```python
from build123d import *

# Parameters (mm, degrees)
BOSS_EXTRUDE1_DEPTH = 6.35
CUT_EXTRUDE1_DEPTH  = 135.362158735
SKETCH3_R           = 1.4732
CUT_EXTRUDE2_DEPTH  = 135.362158735


with BuildPart() as part:
    # Sketch1 → Boss-Extrude1 (new body)
    with BuildSketch(Plane(origin=(0, 0, 0), x_dir=(1, 0, 0), z_dir=(0, 1, 0))):
        with BuildLine():
            Line((0, 0), (114.3, 0))
            ThreePointArc((114.3, 0), (116.096051224, -0.743948776), (116.84, -2.54))
            Line((116.84, -2.54), (116.84, -66.04))
            Line((116.84, -66.04), (97.79, -66.04))
            Line((97.79, -66.04), (97.79, -19.05))
            Line((97.79, -19.05), (0, -19.05))
            Line((0, -19.05), (0, 0))
        make_face()
    extrude(amount=BOSS_EXTRUDE1_DEPTH)

    # Sketch2 → Cut-Extrude1 (cut, through all)
    with BuildSketch(Plane(origin=(0, 6.35, 0), x_dir=(1, 0, 0), z_dir=(0, 1, 0))):
        Polygon((14.533087105, -12.7), (16.366174209, -9.525), (14.533087105, -6.35), (10.866912895, -6.35), (9.033825791, -9.525), (10.866912895, -12.7), align=None)
    extrude(amount=-CUT_EXTRUDE1_DEPTH, mode=Mode.SUBTRACT)

    # Sketch3 → Cut-Extrude2 (cut, through all)
    with BuildSketch(Plane.XZ):
        with Locations(Location((110.49, 38.1, 0), (0, 0, 270))):
            Circle(SKETCH3_R)
        with Locations(Location((110.49, 12.7, 0), (0, 0, 270))):
            Circle(SKETCH3_R)
    extrude(amount=-CUT_EXTRUDE2_DEPTH, mode=Mode.SUBTRACT)


solid = part.part
```
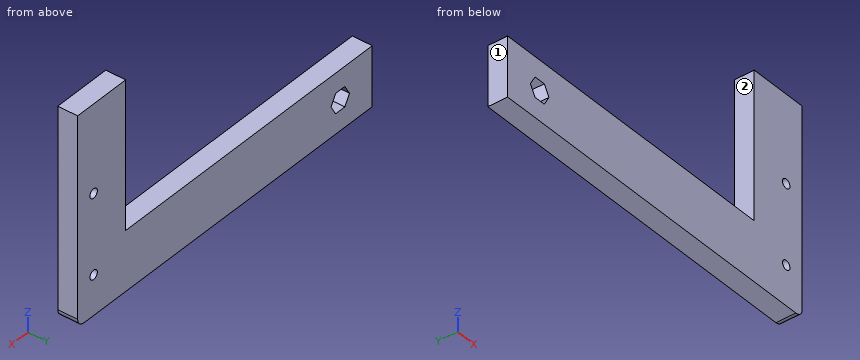
Source: CAD feature listing. Evaluate the final solid. Frame: model axes, mm. Face numbers are marked on the shaded views. A direction names the side the tool comes from. Give positions to 0.01 mm unless a question says otherwise; leave off trailing zeros. Order: outer loops, then holes, each group sorted by start corner. A loop starts at its lowest first (then second) coordinate and runs counter-clockwise, first axis right, second up. Notation, with made-up numbers: (4.5, 8.25) -> (60.5, 8.25) arc R10 ccw to (60.5, 18.25) -> close; hole circle Ø11 at (-5.5, 81). An arc over 180 degrees is marked (long way). Use a Markdown table: item, result.
Q1. First-contact query: P1, Ø3, axis at x = 30.5, y = 3.5, coming from the +Z side. Flat tip, straight axial feed; report the tip coordinate or a pass-through.
A:
| item | result |
|---|---|
| P1 | z = 19.05 |
Q2. Material intervals for line 1 (Z direction, x = 110.49, y = 2.25); line 2 (X direction, y = 5, z = 38.1); line 3 (Z direction, x = 18.5, y = 3), sorted ascending. Write a range as [from, to].
A:
| item | result |
|---|---|
| line 1 | [0, 11.23], [14.17, 36.63], [39.57, 66.04] |
| line 2 | [97.79, 109.02], [111.96, 116.84] |
| line 3 | [0, 19.05] |
Q3. Section C-C (y = 3). Return the cut outline in (x, z) (3 decimals).
A:
| item | result |
|---|---|
| outline | (0, 0) -> (114.3, 0) arc R2.54 ccw to (116.84, 2.54) -> (116.84, 66.04) -> (97.79, 66.04) -> (97.79, 19.05) -> (0, 19.05) -> close; hole (9.034, 9.525) -> (10.867, 6.35) -> (14.533, 6.35) -> (16.366, 9.525) -> (14.533, 12.7) -> (10.867, 12.7) -> close; hole circle Ø2.946 at (110.49, 12.7); hole circle Ø2.946 at (110.49, 38.1) |
Q4. Section D-D (x = 66). Return the cut outline in (y, z).
A:
| item | result |
|---|---|
| outline | (0, 0) -> (6.35, 0) -> (6.35, 19.05) -> (0, 19.05) -> close |
Q5. Access query for the marked faces 1 and 2. Directions: +Z, -Z, +X, -X, +Y, -Y. A direction counts if a zero-diameter tool reaches every point of the face in a straight line with its end or side. Return the directions, or none.
A:
| item | result |
|---|---|
| face 1 | +Z, -Z, -X, +Y, -Y |
| face 2 | +Z, -X, +Y, -Y |
Q6. Section B-B (x = 110.49). Return the cut outline in (y, z), and give its area (3 significant figures).
A:
| item | result |
|---|---|
| outline | (0, 0) -> (6.35, 0) -> (6.35, 11.23) -> (0, 11.23) -> close; (0, 14.17) -> (6.35, 14.17) -> (6.35, 36.63) -> (0, 36.63) -> close; (0, 39.57) -> (6.35, 39.57) -> (6.35, 66.04) -> (0, 66.04) -> close |
| area | 382 mm^2 |
Q7. Section A-A (z = 38.1). Return the cut outline in (x, y).
A:
| item | result |
|---|---|
| outline | (97.79, 0) -> (109.02, 0) -> (109.02, 6.35) -> (97.79, 6.35) -> close; (111.96, 0) -> (116.84, 0) -> (116.84, 6.35) -> (111.96, 6.35) -> close |
